```python
from build123d import *

# Parameters (mm, degrees)
SKETCH2_R          = 1
CUT_EXTRUDE1_DEPTH = 0.3
CHAMFER1_SIZE      = 0.3
SKETCH3_R          = 1
CUT_EXTRUDE2_DEPTH = 0.7


with BuildPart() as part:
    # Sketch1 → Revolve1 (revolve)
    with BuildSketch(Plane(origin=(0, 0, 0), x_dir=(1, 0, 0), z_dir=(0, 1, 0)), mode=Mode.PRIVATE) as revolve1_sk:
        Polygon((0, 0), (0, 2.5), (-3, 2.5), (-3, 3), (-2, 4), (0.5, 4), (4, 1.979274058), (4, 0), align=None)
    revolve(revolve1_sk.sketch.rotate(Axis((-1.085106383, 0, 0), (1, 0, 0)), 180), axis=Axis((-1.085106383, 0, 0), (1, 0, 0)))

    # Sketch2 → Cut-Extrude1 (cut)
    with BuildSketch(Plane(origin=(4, 0, 0), x_dir=(0, 0, -1), z_dir=(1, 0, 0))):
        Circle(SKETCH2_R)
    extrude(amount=-CUT_EXTRUDE1_DEPTH, mode=Mode.SUBTRACT)

    # Chamfer1
    chamfer1_edges = [part.edges().sort_by_distance(p)[0] for p in [
        (4, 0, 1),
    ]]
    chamfer(chamfer1_edges, length=CHAMFER1_SIZE - 0.0001)  # a hair under: the kernel refuses the full size

    # Sketch3 → Cut-Extrude2 (cut)
    with BuildSketch(Plane(origin=(3.7, 0, 0), x_dir=(0, 0, -1), z_dir=(1, 0, 0))):
        Circle(SKETCH3_R)
    extrude(amount=-CUT_EXTRUDE2_DEPTH, mode=Mode.SUBTRACT)

    # Cut-Extrude3 cone 1 section (through the dimple's axis) → Cut-Extrude3 (revolve, cut)
    with BuildSketch(Plane(origin=(3, 0, 0), x_dir=(0, 0, -1), z_dir=(0, 1, 0))):
        Polygon((0, 0), (1, 0), (0, 1), align=None)
    revolve(axis=Axis((3, 0, 0), (-1, 0, 0)), mode=Mode.SUBTRACT)


solid = part.part
```
Design review of the part built by this model. Coordinates are the model's own, in mm. A direction names the side the tool comes from. Round coordinates to 2 decimals unless told otherwise and drop trailing zeros. Write each loop counter-clockwise with the first axis right and the second up, starting at its lowest first coordinate (ties: lowest second). Pieces come first, ordered by that corner, then holes.
Item 1: Clearance check with flat-ended pins moving along their axes: pin 1 Ø1.5 at (x, y) = (0.5, -2.5) entering from +Z; pin 2 Ø4 at (x, z) = (-1.5, -0.5) entering from +Y; pin 3 Ø1.8 at (y, z) = (0, 0) entering from +X; pin 4 Ø1 at (x, y) = (1.5, -2) entering from +Z. State where each tip first meets the part, or that it passes through.
Item 2: For probe 1 along X at (y, z) = (1, -1.25); probe 2 along Y at (x, z) = (-1.25, 0); probe 3 along Z at (x, y) = (-0.5, -1.5), list the stretches that pass through material, from the lowest coordinate up.
Item 3: The part is to be moulded in two halves that separate along Y. For faces 3 (the conical face through (2, 0, 0)), 4 (the cylindrical face through (-0.732, 3.905, -0.867)), 5 (the flat face through (-3, -2, 2)), say which applies: +Y half, -Y half, draft (parallel to the pull), parting line (faces both ways), or undercut.
Item 4: We need section A-A on x = -1.25. Write out the cut boundary in (y, z), and give its area (3 significant figures).
Item 5: We need section B-B on x = 1.25. Write out the cut boundary in (y, z), and give its area (3 significant figures).
Item 6: For faces 1 (the cylindrical face through (3.355, -0.976, 0.217)), 2 (the flat face through (0, 0, 0)), list the 3-axis set-ups (+Z, -Z, +X, -X, +Y, -Y) from which the entire face can be reached by the end or side of a thin tool; tool diameter is ignored.
Returned:
1. pin 1: stops at z = 3.6
1. pin 2: stops at y = 4
1. pin 3: stops at x = 2.9
1. pin 4: stops at z = 3.23
2. probe 1: x = 0 to 4
2. probe 2: y = -4 to -2.5, 2.5 to 4
2. probe 3: z = -3.71 to -2, 2 to 3.71
3. face 3: undercut
3. face 4: parting line
3. face 5: draft
4. outline: circle Ø8 at (0, 0); hole circle Ø5 at (0, 0)
4. area: 30.6 mm2
5. outline: circle Ø7.13 at (0, 0)
5. area: 40.0 mm2
6. face 1: +X
6. face 2: -X
